Verification items for the finished model (mm, model axes). A direction names the side the tool comes from. Round coordinates to 2 decimals unless told otherwise and drop trailing zeros. Write each loop counter-clockwise with the first axis right and the second up, starting at its lowest first coordinate (ties: lowest second). Pieces come first, ordered by that corner, then holes. Notation, with made-up numbers: M -28.75,83.5 L 2.25,83.5 A27 cw 2.25,114.5 Z; hole C -24,12.5 d1. An arc over 180 degrees is marked long. One line per question, with ' | ' between items. Start each with the question number.
Q1. Tool access check on faces 4 (the face through (0, 7, 5.1)), 5 (the face through (0, 0, 0)). Record the directions out of +Z, -Z, +X, -X, +Y, -Y that give a thin tool (end or side, any length) a straight path to the whole face; none if there is none.
Q2. Cross-section at A-A (y = 10.5). Record the boundary of the cut face in (x, z), then the cut area to 3 significant figures.
Q3. Release check for a two-part mould opening along Z. For faces 1 (the face through (0.1, 12.53, -4.95)), 2 (the face through (-7.2, 5, 0)), 3 (the face through (0, 7, 7.5)) record: released by +Z, released by -Z, zero draft, split by the parting line, or undercut.
Q4. Thickness scan on line 1 along Y through (x, z) = (3.25, 3.5); line 2 along Y through (x, z) = (6, 0.5); line 3 along Z through (x, y) = (4.75, 0.5). Record the ranges inside material, lowest first. Write a range as from..to.
Q5. Cross-section at B-B (y = 12.25). Record the boundary of the cut face in (x, z), then the cut area to 3 significant figures.
Q6. Gauge pin test, flat ends, axial feed: pin 1 (2 mm diameter, centred on x = -5, z = -3.5, fed in from +Y); pin 2 (6 mm diameter, centred on x = -4.5, z = -6, fed in from +Y). Record the tip position at first contact, or that the pin passes through.
Q7. Cross-section at C-C (z = 3.25). Record the boundary of the cut face in (x, y), then the cut area to 3 significant figures.
from build123d import *

# Parameters (mm, degrees)
SKIZZE1_W                       = 14.4
SKIZZE1_H                       = 15
AUFSATZ_LINEAR_AUSTRAGEN1_DEPTH = 13
SKIZZE2_W                       = 14.4
SKIZZE2_H                       = 1
SCHNITT_LINEAR_AUSTRAGEN1_DEPTH = 11
VERRUNDUNG1_R                   = 1
FASE1_SIZE                      = 2
VERRUNDUNG3_R                   = 0.5


# Some blends are built 0.0001 mm under size
with BuildPart() as part:
    # Skizze1 → Aufsatz-Linear austragen1 (new body)
    with BuildSketch(Plane(origin=(0, 0, 0), x_dir=(1, 0, 0), z_dir=(0, 1, 0))):
        Rectangle(SKIZZE1_W, SKIZZE1_H)
    extrude(amount=AUFSATZ_LINEAR_AUSTRAGEN1_DEPTH)

    # Skizze2 → Schnitt-Linear austragen1 (cut)
    with BuildSketch(Plane(origin=(0, 13, 0), x_dir=(1, 0, 0), z_dir=(0, 1, 0))):
        with Locations((0, -5.6)):
            Rectangle(SKIZZE2_W, SKIZZE2_H)
        with Locations((0, -3.5)):
            Rectangle(SKIZZE2_W, SKIZZE2_H)
        with Locations((0, -1.4)):
            Rectangle(SKIZZE2_W, SKIZZE2_H)
        with Locations((0, 1.4)):
            Rectangle(SKIZZE2_W, SKIZZE2_H)
        with Locations((0, 3.5)):
            Rectangle(SKIZZE2_W, SKIZZE2_H)
        with Locations((0, 5.6)):
            Rectangle(SKIZZE2_W, SKIZZE2_H)
    extrude(amount=-SCHNITT_LINEAR_AUSTRAGEN1_DEPTH, mode=Mode.SUBTRACT)

    # Verrundung1
    # the kernel refuses this fillet: 1 mm, written as the material it takes off along each edge
    with BuildSketch(Plane(origin=(-9.7, 13, 7.5), x_dir=(0, -1, 0), z_dir=(1, 0, 0)), Plane(origin=(-9.7, 13, 6.1), x_dir=(0, 0, 1), z_dir=(1, 0, 0)), Plane(origin=(-9.7, 13, 3), x_dir=(0, -1, 0), z_dir=(1, 0, 0)), Plane(origin=(-9.7, 13, 0.9), x_dir=(0, -1, 0), z_dir=(1, 0, 0)), Plane(origin=(-9.7, 13, -1.9), x_dir=(0, -1, 0), z_dir=(1, 0, 0)), Plane(origin=(-9.7, 13, -4), x_dir=(0, -1, 0), z_dir=(1, 0, 0)), Plane(origin=(-9.7, 13, -6.1), x_dir=(0, -1, 0), z_dir=(1, 0, 0))) as verrundung1_piece_1:
        with BuildLine():
            CenterArc((VERRUNDUNG1_R, VERRUNDUNG1_R), VERRUNDUNG1_R, 180, 90)
            Line((0, VERRUNDUNG1_R), (0, 0))
            Line((0, 0), (VERRUNDUNG1_R, 0))
        make_face()
    extrude(amount=19.4, mode=Mode.SUBTRACT)
    with BuildSketch(Plane(origin=(9.7, 13, 5.1), x_dir=(0, -1, 0), z_dir=(-1, 0, 0)), Plane(origin=(9.7, 13, 4), x_dir=(0, 0, 1), z_dir=(-1, 0, 0)), Plane(origin=(9.7, 13, 1.9), x_dir=(0, 0, 1), z_dir=(-1, 0, 0)), Plane(origin=(9.7, 13, -0.9), x_dir=(0, 0, 1), z_dir=(-1, 0, 0)), Plane(origin=(9.7, 13, -3), x_dir=(0, 0, 1), z_dir=(-1, 0, 0)), Plane(origin=(9.7, 13, -5.1), x_dir=(0, 0, 1), z_dir=(-1, 0, 0)), Plane(origin=(9.7, 13, -7.5), x_dir=(0, 0, 1), z_dir=(-1, 0, 0))) as verrundung1_piece_2:
        with BuildLine():
            CenterArc((VERRUNDUNG1_R, -VERRUNDUNG1_R), VERRUNDUNG1_R, 90, 90)
            Line((0, -VERRUNDUNG1_R), (0, 0))
            Line((0, 0), (VERRUNDUNG1_R, 0))
        make_face()
    extrude(amount=19.4, mode=Mode.SUBTRACT)

    # Fase1
    fase1_edges = [part.edges().sort_by_distance(p)[0] for p in [
        (0, 0, 7.5),
        (0, 0, -7.5),
    ]]
    chamfer(fase1_edges, length=FASE1_SIZE)

    # Verrundung3
    verrundung3_edges = [part.edges().sort_by_distance(p)[0] for p in [
        (0, 2, -5.1),
        (0, 2, -3),
        (0, 2, -0.9),
        (0, 2, 1.9),
        (0, 2, 4),
        (0, 2, 6.1),
        (0, 2, 5.1),
        (0, 2, 3),
        (0, 2, 0.9),
        (0, 2, -1.9),
        (0, 2, -4),
        (0, 2, -6.1),
    ]]
    fillet(verrundung3_edges, radius=VERRUNDUNG3_R - 0.0001)  # a hair under: the kernel refuses the full size


solid = part.part
Determined:
1) face 4: +X, -X, +Y | face 5: +Z, -Z, +X, -X, -Y
2) outline: M -7.2,-7.5 L 7.2,-7.5 L 7.2,-6.1 L -7.2,-6.1 Z; M -7.2,-5.1 L 7.2,-5.1 L 7.2,-4 L -7.2,-4 Z; M -7.2,-3 L 7.2,-3 L 7.2,-1.9 L -7.2,-1.9 Z; M -7.2,-0.9 L 7.2,-0.9 L 7.2,0.9 L -7.2,0.9 Z; M -7.2,1.9 L 7.2,1.9 L 7.2,3 L -7.2,3 Z; M -7.2,4 L 7.2,4 L 7.2,5.1 L -7.2,5.1 Z; M -7.2,6.1 L 7.2,6.1 L 7.2,7.5 L -7.2,7.5 Z | area: 130 mm²
3) face 1: undercut | face 2: zero draft | face 3: released by +Z
4) line 1: y = 0..2 | line 2: y = 0..12.8 | line 3: z = -6..6
5) outline: M -7.2,-7.47 L 7.2,-7.47 L 7.2,-6.13 L -7.2,-6.13 Z; M -7.2,-5.07 L 7.2,-5.07 L 7.2,-4.03 L -7.2,-4.03 Z; M -7.2,-2.97 L 7.2,-2.97 L 7.2,-1.93 L -7.2,-1.93 Z; M -7.2,-0.87 L 7.2,-0.87 L 7.2,0.87 L -7.2,0.87 Z; M -7.2,1.93 L 7.2,1.93 L 7.2,2.97 L -7.2,2.97 Z; M -7.2,4.03 L 7.2,4.03 L 7.2,5.07 L -7.2,5.07 Z; M -7.2,6.13 L 7.2,6.13 L 7.2,7.47 L -7.2,7.47 Z | area: 123 mm²
6) pin 1: stops at y = 12.87 | pin 2: stops at y = 12.95
7) outline: M -7.2,0 L 7.2,0 L 7.2,2.07 L -7.2,2.07 Z | area: 29.8 mm²
